Print and shaded views of the part. All mm, measured from the part's lowest x, y and z. A direction names the side the tool comes from. Give positions to 0.01 mm unless a question says otherwise; leave off trailing zeros. Write each loop counter-clockwise with the first axis right and the second up, starting at its lowest first coordinate (ties: lowest second). Pieces come first, ordered by that corner, then holes. Notation, with made-up numbers: M 82.25,-9.5 L 128.25,-9.5 A3 ccw 128.25,-4.5 Z; hole C -16.75,37 d2. An arc over 180 degrees is marked long. One line per question, with ' | ' between items. Start each with the question number.
1. Cut at B-B, the plane y = 3.75. Write the cut outline in (x, z), then the cut area to 3 significant figures.
2. Flat gauge pin, fed straight in: pin 1 (3 mm diameter, centred on x = 3, z = 9.5, fed in from +Y). Where does the tip first touch, or does it go through?
3. Cut at D-D, the plane z = 10. Write the cut outline in (x, y), then the cut area to 3 significant figures.
4. Wall check: L1, parallel to Y at x = 1.75, z = 11.5; L2, parallel to Z at x = 5.2, y = 2.25; L3, parallel to X at y = 3.8, z = 10. Give the ranges that are in metal, low to high.
5. Cut at C-C, the plane x = 3.1. Write the cut outline in (y, z).
6. Which spindle directions (+Z, -Z, +X, -X, +Y, -Y) get a long thin tool onto all of the face, cutting with end or side? Do the marked faces 1 and 2. Say none if no direction does.
7. Cut at A-A, the plane x = 5.5. Write the cut outline in (y, z), then the cut area to 3 significant figures.
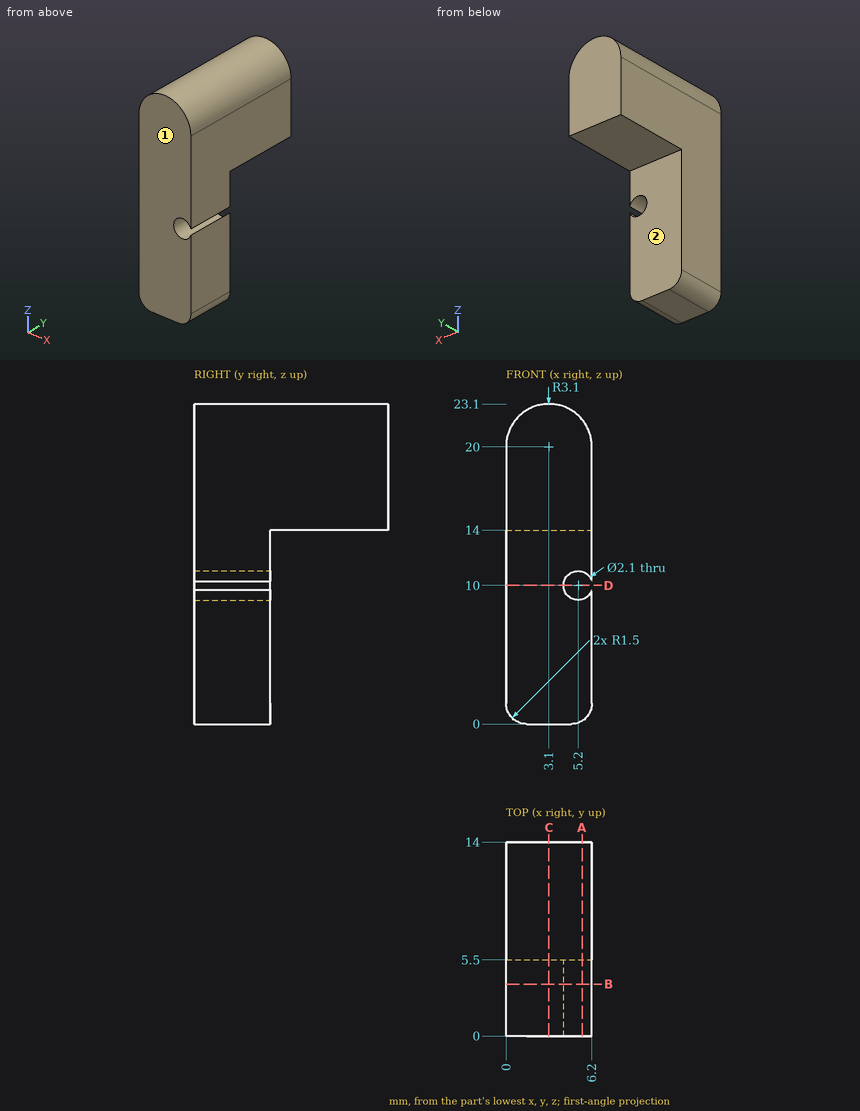
Here are the results:
1) outline: M 0,1.5 A1.5 ccw 1.5,0 L 4.7,0 A1.5 ccw 6.2,1.5 L 6.2,9.68 A1.05 cw long 6.2,10.32 L 6.2,20 A3.1 ccw 0,20 Z | area: 135 mm^2
2) pin 1: y = 5.5
3) outline: M 0,0 L 4.15,0 L 4.15,5.5 L 0,5.5 Z | area: 22.8 mm^2
4) L1: 0 to 5.5 | L2: 0.09 to 8.95, 11.05 to 22.28 | L3: 0 to 4.15
5) outline: M 0,0 L 5.5,0 L 5.5,14 L 14,14 L 14,23.1 L 0,23.1 Z
6) face 1: +Z, -Z, +X, -X, -Y | face 2: -Z, +X, -X, +Y
7) outline: M 0,0.23 L 5.5,0.23 L 5.5,8.99 L 0,8.99 Z; M 0,11.01 L 5.5,11.01 L 5.5,14 L 14,14 L 14,21.96 L 0,21.96 Z | area: 176 mm^2
